Autodesk Inventor part; units mm, degrees
ref_plane "YZ Plane" through (0, 0, 0) normal (1, 0, 0) x (0, 1, 0)
ref_plane "XZ Plane" through (0, 0, 0) normal (0, 1, 0) x (-1, 0, 0)
ref_plane "XY Plane" through (0, 0, 0) normal (0, 0, 1) x (1, 0, 0)
sketch "Эскиз1" plane through (0, 0, 0) normal (0, 1, 0) x (-1, 0, 0)
  line L0 (-14.9924, 37.5) -> (15.0076, 37.5)
  line L1 (15.0076, 37.5) -> (15.0076, -17.5)
  line L2 (15.0076, -17.5) -> (-14.9924, -17.5)
  line L3 (-14.9924, -17.5) -> (-14.9924, 37.5)
  circle A0 centre (0, -10) radius 4.1
  circle A1 centre (0, 10) radius 4.1
  line L4 (15.0076, -17.5) -> (-14.9924, -17.5)
  line L5 (-14.9924, -17.5) -> (-14.9924, -40.5)
  line L6 (-14.9924, -40.5) -> (15.0076, -40.5)
  line L7 (15.0076, -40.5) -> (15.0076, -17.5)
  point P0 (0, 0)
  dimension "d0" = 30
  dimension "d1" = 55
  dimension "d2" = 8.2
  dimension "d3" = 8.2
  dimension "d4" = 10
  dimension "d5" = 10
  dimension "d11" = 23
extrude "Выдавливание1" add sketch "Эскиз1" along normal blind 5
sketch "Эскиз4" plane through (0, 5, 0) normal (0, 1, 0) x (1, 0, 0)
  line L0 (14.9924, -37.5) -> (-15.0076, -37.5)
  line L1 (-0.0076, -37.5) -> (-0.0076, -22.5)
  line L2 (8.9924, -37.5) -> (-9.0076, -37.5)
  line L3 (-9.0076, -37.5) -> (-9.0076, -22.5)
  line L4 (-9.0076, -22.5) -> (8.9924, -22.5)
  line L5 (8.9924, -22.5) -> (8.9924, -37.5)
  line L6 (8.9924, -37.5) -> (-9.0076, -22.5) construction
  line L7 (-9.0076, -37.5) -> (8.9924, -22.5) construction
  point P0 (0, 0)
  point P1 (-0.0076, -30)
  dimension "d19" = 15
  dimension "d20" = 18
  dimension "d21" = 15
extrude "Выдавливание4" add sketch "Эскиз4" along normal blind 15
sketch "Эскиз5" plane through (8.9924, 5, 37.5) normal (1, 0, 0) x (0, 0, -1)
  line L0 (0, 15) -> (15, 15)
  line L1 (7.5, 15) -> (7.5, 0)
  line L2 (78, 0) -> (0, 0)
  circle A0 centre (7.5, 7.5) radius 3
  point P0 (37.5, -5)
  dimension "d24" = 6
extrude "Выдавливание5" cut sketch "Эскиз5" against normal blind 20
fillet "Сопряжение1" radius 7.5 2 edges at (-0.0076, 20, 22.5) (-0.0076, 20, 37.5)
sketch "Эскиз6" plane through (0, 5, 0) normal (0, 1, 0) x (1, 0, 0)
  line L0 (14.9924, 40.5) -> (-15.0076, 40.5)
  line L1 (-0.0076, 40.5) -> (-0.0076, 35.5)
  circle A0 centre (-0.0076, 35.5) radius 1.75
  point P0 (0, 0)
  dimension "d28" = 5
  dimension "d29" = 3.5
extrude "Выдавливание6" cut sketch "Эскиз6" against normal blind 15
sketch "Эскиз7" plane through (0, 5, 0) normal (0, 1, 0) x (1, 0, 0)
  circle A0 centre (0, -10) radius 4.1
  circle A1 centre (0, -10) radius 7.5
  circle A2 centre (0, 10) radius 4.1
  circle A3 centre (0, 10) radius 7.5
  point P0 (0, 0)
  dimension "d32" = 15
  dimension "d33" = 15
extrude "Выдавливание7" cut sketch "Эскиз7" against normal blind 3
properties part number "КВ33.044.601 - Опора держателя катка"
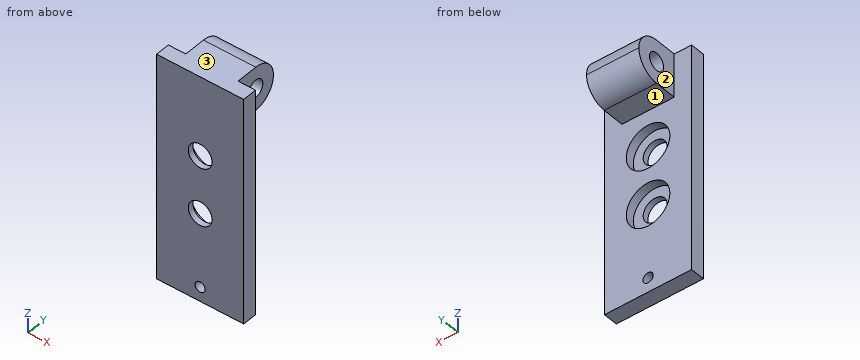
Can you work these out from the model? Positions are in its coordinate system, mm. Face numbers are marked on the shaded views. A direction names the side the tool comes from. Give positions to 0.01 mm unless a question says otherwise; leave off trailing zeros. Write each loop counter-clockwise with the first axis right and the second up, starting at its lowest first coordinate (ties: lowest second). Pieces come first, ordered by that corner, then holes. Notation, with made-up numbers: M 76,51 L 102,51 A15 ccw 102,57 Z; hole C 61,70 d4. An arc over 180 degrees is marked long. Answer in a Markdown table with one row per item. Add a question column.
Item 1: Imagine slicing it at B-B, the plane z = 10. Write out the boundary of the cut face in (x, y).
Item 2: Imagine slicing it at A-A, the plane x = 0. State how many separate pieces and enclosed holes the cut face has, plus the area to 3 significant figures.
Item 3: On a 3-axis mill with a long thin cutter (end or side, diameter ignored), from which of +Z, -Z, +X, -X, +Y, -Y can I reach the whole of each face in a straight line? I mean the marked faces 1, 2 and 3. Say none if no direction works.
Item 4: Please list where these lines run through material, in increasing order: L1, parallel to Z at x = 0, y = 0.5; L2, parallel to X at y = 1.65, z = -35.5; L3, parallel to X at y = 3.3, z = 10.
Item 5: Imagine slicing it at D-D, the plane z = -35.5. Write out the boundary of the cut face in (x, y), plus the area to 4 significant figures.
Item 6: For pin 1 Ø12 at (x, z) = (0, 10) entering from +Y; pin 2 Ø8 at (y, z) = (12.5, 30) entering from -X; pin 3 Ø4 at (x, y) = (5, 15.5) entering from -Z, each with a flat end and sliding along its axis, tell me the tip position at first contact or that it passes through.
Evaluation:
| question | item | result |
|---|---|---|
| 1 | outline | M -15.01,0 L -4.1,0 L -4.1,2 L -7.5,2 L -7.5,5 L -15.01,5 Z; M 4.1,0 L 14.99,0 L 14.99,5 L 7.5,5 L 7.5,2 L 4.1,2 Z |
| 2 | separate pieces | 4 |
| 2 | enclosed holes | 1 |
| 2 | area | 422 mm² |
| 3 | face 1 | -Z, +X, -X, +Y |
| 3 | face 2 | +Z, -Z, -X, +Y |
| 3 | face 3 | +Z, +X, -X, +Y, -Y |
| 4 | L1 | z = -40.5 to -37.25, -33.75 to -14.1, -5.9 to 5.9, 14.1 to 37.5 |
| 4 | L2 | x = -15.01 to -1.76, 1.74 to 14.99 |
| 4 | L3 | x = -15.01 to -7.5, 7.5 to 14.99 |
| 5 | outline | M -15.01,0 L -1.76,0 L -1.76,5 L -15.01,5 Z; M 1.74,0 L 14.99,0 L 14.99,5 L 1.74,5 Z |
| 5 | area | 132.5 mm² |
| 6 | pin 1 | stops at y = 2 |
| 6 | pin 2 | stops at x = -9.01 |
| 6 | pin 3 | stops at z = 22.57 |
